Here's how the part is built. I have some questions about the finished solid (model axes, mm). A direction names the side the tool comes from. Give positions to 0.01 mm unless a question says otherwise; leave off trailing zeros. Order: outer loops, then holes, each group sorted by start corner. A loop starts at its lowest first (then second) coordinate and runs counter-clockwise, first axis right, second up.
from build123d import *

# Parameters (mm, degrees)
SKETCH1_W           = 24.7
SKETCH1_H           = 7.7
BOSS_EXTRUDE1_DEPTH = 10
CUT_EXTRUDE1_DEPTH  = 10
SKETCH3_W           = 5
SKETCH3_H           = 6
CUT_EXTRUDE2_DEPTH  = 10
SKETCH4_W           = 3
SKETCH4_H           = 7.7
BOSS_EXTRUDE2_DEPTH = 3


with BuildPart() as part:
    # Sketch1 → Boss-Extrude1 (new body)
    with BuildSketch(Plane.XY):
        Rectangle(SKETCH1_W, SKETCH1_H)
    extrude(amount=BOSS_EXTRUDE1_DEPTH)

    # Sketch2 → Cut-Extrude1 (cut)
    with BuildSketch(Plane.XZ.offset(3.85)):
        Polygon((4.4, 5), (2.2, 8.810511777), (-2.2, 8.810511777), (-4.4, 5), (-2.2, 1.189488223), (2.2, 1.189488223), align=None)
    extrude(amount=-CUT_EXTRUDE1_DEPTH, mode=Mode.SUBTRACT)

    # Sketch3 → Cut-Extrude2 (cut)
    with BuildSketch(Plane(origin=(0, 3.85, 0), x_dir=(1, 0, 0), z_dir=(0, 1, 0))):
        with Locations((-7.85, -5)):
            Rectangle(SKETCH3_W, SKETCH3_H)
    cut_extrude2 = extrude(amount=-CUT_EXTRUDE2_DEPTH, mode=Mode.SUBTRACT)

    # Mirror1: Cut-Extrude2 across plane
    add(cut_extrude2.mirror(Plane(origin=(0, 0, 0), x_dir=(0, 0, 1), z_dir=(1, 0, 0))), mode=Mode.SUBTRACT)

    # Sketch4 → Boss-Extrude2 (add)
    with BuildSketch(Plane(origin=(12.35, 0, 0), x_dir=(0, 0, -1), z_dir=(1, 0, 0))):
        with Locations((-8.5, 0)):
            Rectangle(SKETCH4_W, SKETCH4_H)
    boss_extrude2 = extrude(amount=BOSS_EXTRUDE2_DEPTH)

    # Mirror2: Boss-Extrude2 across plane
    add(boss_extrude2.mirror(Plane(origin=(0, 0, 0), x_dir=(0, 0, 1), z_dir=(1, 0, 0))))


solid = part.part
Q1. If we section it at B-B on y = 1: List the corners of the cut face in (x, z) for me.
Filled sheet:
outline: (-15.35, 7) - (-12.35, 7) - (-12.35, 0) - (12.35, 0) - (12.35, 7) - (15.35, 7) - (15.35, 10) - (-15.35, 10) - close; hole (-10.35, 2) - (-5.35, 2) - (-5.35, 8) - (-10.35, 8) - close; hole (-4.4, 5) - (-2.2, 1.19) - (2.2, 1.19) - (4.4, 5) - (2.2, 8.81) - (-2.2, 8.81) - close; hole (5.35, 2) - (10.35, 2) - (10.35, 8) - (5.35, 8) - close
Q2. If we section it at A-A on x = 1: List the corners of the cut face in (y, z) for me.
Filled sheet:
outline: (-3.85, 0) - (3.85, 0) - (3.85, 1.19) - (-3.85, 1.19) - close; (-3.85, 8.81) - (3.85, 8.81) - (3.85, 10) - (-3.85, 10) - close
Q3. For faces 1 (the face through (-8, 0, 2)), 2 (the face through (-12.35, 0, 3)), 3 (the face through (12.35, 0, 3)), which set-ups out of +Z, -Z, +X, -X, +Y, -Y let a thin tool reach every point of the face, with its end or its side?
Filled sheet:
face 1: +Y, -Y
face 2: -Z, -X, +Y, -Y
face 3: -Z, +X, +Y, -Y
Q4. If we section it at C-C on z = 5.5: List the corners of the cut face in (x, y) for me, plus the area to 3 significant figures.
Filled sheet:
outline: (-12.35, -3.85) - (-10.35, -3.85) - (-10.35, 3.85) - (-12.35, 3.85) - close; (-5.35, -3.85) - (-4.11, -3.85) - (-4.11, 3.85) - (-5.35, 3.85) - close; (4.11, -3.85) - (5.35, -3.85) - (5.35, 3.85) - (4.11, 3.85) - close; (10.35, -3.85) - (12.35, -3.85) - (12.35, 3.85) - (10.35, 3.85) - close
area: 49.9 mm2
Q5. I need wall thicknesses on L1, parallel to Z at x = 10, y = 3; L2, parallel to X at y = -1, z = 6; L3, parallel to X at y = 3, z = 7.25. Which ranges of each line are inside material? Lowest first, please.
Filled sheet:
L1: z = 0 to 2, 8 to 10
L2: x = -12.35 to -10.35, -5.35 to -3.82, 3.82 to 5.35, 10.35 to 12.35
L3: x = -15.35 to -10.35, -5.35 to -3.1, 3.1 to 5.35, 10.35 to 15.35
Q6. If we section it at D-D on x = -6.5: List the corners of the cut face in (y, z) for me, plus the area to 3 significant figures.
Filled sheet:
outline: (-3.85, 0) - (3.85, 0) - (3.85, 2) - (-3.85, 2) - close; (-3.85, 8) - (3.85, 8) - (3.85, 10) - (-3.85, 10) - close
area: 30.8 mm2
Q7. Thinking about a two-plate mould opening in Z: for faces 4 (the face through (3.285, -0.054, 3.068)), 5 (the face through (0, 0, 1.189)), 6 (the face through (15.35, 0, 9)), 7 (the face through (0, 0, 10)), which applies, released by +Z, released by -Z, zero draft, split by the parting line, or undercut?
Filled sheet:
face 4: undercut
face 5: undercut
face 6: zero draft
face 7: released by +Z
Q8. I'm going to push flat-ended pins straight in: P1, Ø0.9, axis at x = 14.5, y = 1.5, coming from the -Z side; P2, Ø3.5, axis at y = 0.5, z = 4, coming from the +X side; P3, Ø3.5, axis at y = 1.5, z = 5, coming from the -X side. Where does each tip first touch, or does it pass through?
Filled sheet:
P1: stops at z = 7
P2: stops at x = 12.35
P3: stops at x = -12.35
